The drawing under review shows one solid part. Ordinate dimensions are in mm from its lowest x, y, z. A direction names the side the tool comes from. Coordinates: 2 decimals unless noted, no trailing zeros. Write each loop counter-clockwise with the first axis right and the second up, starting at its lowest first coordinate (ties: lowest second). Pieces come first, ordered by that corner, then holes.
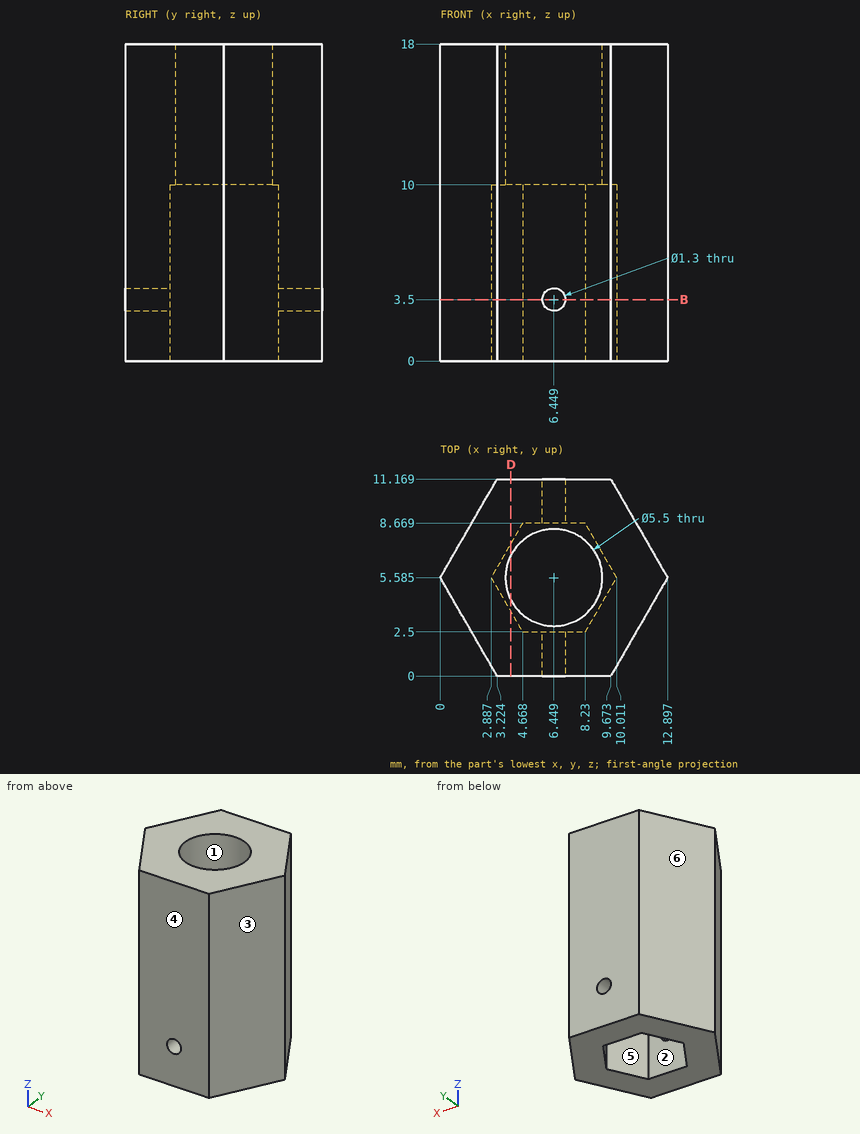
Q1. Tool access review of the marked faces 1 and 2: name each direction out of +Z, -Z, +X, -X, +Y, -Y from which nothing blocks a thin tool from reaching the whole face with its end or side.
Ans:
face 1: +Z, -Z
face 2: -Z
Q2. Draft analysis for pull direction X (two halves, no side actions). For the marked faces 3, 4, 5 and 6, state which applies: +X half, -X half, draft (parallel to the pull), parting line (faces both ways), or undercut.
Ans:
face 3: +X half
face 4: draft
face 5: undercut
face 6: -X half
Q3. Add section D-D (x = 4). State the section outline as (y, z) points.
Ans:
outline: (0, 0) - (3.66, 0) - (3.66, 10) - (4.33, 10) - (4.33, 18) - (0, 18) - close; (6.84, 10) - (7.51, 10) - (7.51, 0) - (11.17, 0) - (11.17, 18) - (6.84, 18) - close
Q4. Add section B-B (z = 3.5). State the section outline as (x, y) points (1 decimal).
Ans:
outline: (0, 5.6) - (3.2, 0) - (5.8, 0) - (5.8, 2.5) - (4.7, 2.5) - (2.9, 5.6) - (4.7, 8.7) - (5.8, 8.7) - (5.8, 11.2) - (3.2, 11.2) - close; (7.1, 0) - (9.7, 0) - (12.9, 5.6) - (9.7, 11.2) - (7.1, 11.2) - (7.1, 8.7) - (8.2, 8.7) - (10, 5.6) - (8.2, 2.5) - (7.1, 2.5) - close
Q5. For probe 1 along Z at (x, y) = (8, 8.5); probe 2 along X at (y, z) = (9.85, 3.5) (1 decimal); probe 3 along Y at (x, z) = (3.75, 4.75) (1 decimal), list the stretches that pass through material, from the lowest coordinate up.
Ans:
probe 1: z = 10 to 18
probe 2: x = 2.5 to 5.8, 7.1 to 10.4
probe 3: y = 0 to 4.1, 7.1 to 11.2
Q6. Clearance check with flat-ended pins moving along their axes: pin 1 Ø2 at (y, z) = (5, 13) entering from -X; pin 2 Ø1 at (y, z) = (2.5, 13.5) entering from -X; pin 3 Ø1.5 at (y, z) = (7, 13.5) entering from +X. State where each tip first meets the part, or that it passes through.
Ans:
pin 1: stops at x = 0
pin 2: stops at x = 1.49
pin 3: stops at x = 12.51
